The figure shows three views and two pictorial views of one solid part (mm, origin at its lowest corner). Answer the questions. Round coordinates to 2 decimals unless told otherwise and drop trailing zeros. Write each loop counter-clockwise with the first axis right and the second up, starting at its lowest first coordinate (ties: lowest second). Pieces come first, ordered by that corner, then holes. Notation, with made-up numbers: (58, -13) -> (87, -13) arc R24 cw to (87, 2) -> close; hole circle Ø11 at (10.5, 12.5). An arc over 180 degrees is marked (long way). One line per item, written item: value.
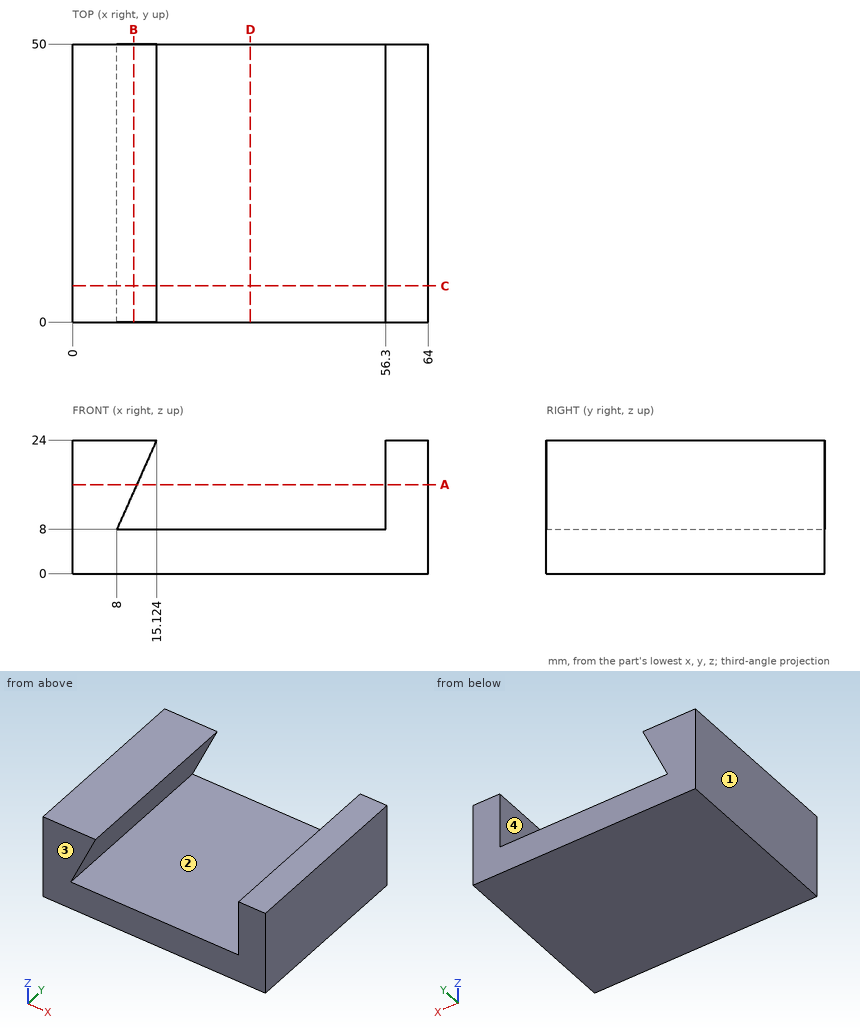
(1) For a pull along X with two mould halves and no side action, classify the marked faces 1, 2, 3 and 4 as pulls with the +X half, pulls with the -X half, needs draft (parallel to the pull), parting line crosses it, or undercut.
Reported:
face 1: pulls with the -X half
face 2: undercut
face 3: needs draft
face 4: undercut
(2) Find section C-C on y = 6.5. Give the vertices of the cut face in (x, z).
Reported:
outline: (0, 0) -> (64, 0) -> (64, 24) -> (56.3, 24) -> (56.3, 8) -> (8, 8) -> (15.12, 24) -> (0, 24) -> close
(3) Find section A-A on z = 16. Give the vertices of the cut face in (x, y).
Reported:
outline: (0, 0) -> (11.56, 0) -> (11.56, 50) -> (0, 50) -> close; (56.3, 0) -> (64, 0) -> (64, 50) -> (56.3, 50) -> close
(4) A flat-ended cylindrical pin translates along its axis: pin 1 Ø1.5 at (x, z) = (35, 9) entering from +Y. Find the tip coordinate at first contact, or state that the pin passes through.
Reported:
pin 1: passes through
(5) Find section D-D on x = 32. Give the vertices of the cut face in (y, z), plus the area to 3 significant figures.
Reported:
outline: (0, 0) -> (50, 0) -> (50, 8) -> (0, 8) -> close
area: 400 mm2
(6) Consider probe 1 along Z at (x, y) = (17.5, 37.5); probe 2 along X at (y, z) = (29.5, 8.5); probe 3 along X at (y, z) = (3.5, 14.5) (1 decimal). Determine where each line is inside the solid, lowest interval first.
Reported:
probe 1: z = 0 to 8
probe 2: x = 0 to 8.22, 56.3 to 64
probe 3: x = 0 to 10.9, 56.3 to 64
(7) Find section B-B on x = 11. Give the vertices of the cut face in (y, z), plus the area to 3 significant figures.
Reported:
outline: (0, 0) -> (50, 0) -> (50, 8) -> (0, 8) -> close; (0, 14.74) -> (50, 14.74) -> (50, 24) -> (0, 24) -> close
area: 863 mm2
